Design review of the part built by this model. Coordinates are the model's own, in mm. A direction names the side the tool comes from. Round coordinates to 2 decimals unless told otherwise and drop trailing zeros. Order: outer loops, then holes, each group sorted by start corner. A loop starts at its lowest first (then second) coordinate and runs counter-clockwise, first axis right, second up. Notation, with made-up numbers: (11, 62.25) - (70, 62.25) arc R16 ccw to (70, 72.25) - close; hole circle Ø1 at (86.25, 35). An arc over 180 degrees is marked (long way). Write item = value, one per line.
from build123d import *

# Parameters (mm, degrees)
BOSS_EXTRUDE1_DEPTH        = 6.35
BOSS_EXTRUDE2_DEPTH        = 6.35
CUT_EXTRUDE2_REACH         = 178.705
SKETCH3_R                  = 25.4
SKETCH3_R_2                = 14.2875
F_6_CLEARANCE_HOLE1_D      = 3.6576
TAP_DRILL_FOR_10_32_TAP1_D = 4.0386


with BuildPart() as part:
    # Sketch1 → Boss-Extrude1 (new body)
    with BuildSketch(Plane(origin=(0, 0, 0), x_dir=(1, 0, 0), z_dir=(0, 1, 0))):
        with BuildLine():
            Line((-82.55, -50.8), (-10.295626201, -150.844517568))
            ThreePointArc((-10.295626201, -150.844517568), (0, -156.108787534), (10.295626201, -150.844517568))
            Line((10.295626201, -150.844517568), (82.55, -50.8))
            Line((82.55, -50.8), (82.55, 50.8))
            Line((82.55, 50.8), (-82.55, 50.8))
            Line((-82.55, 50.8), (-82.55, -50.8))
        make_face()
    extrude(amount=BOSS_EXTRUDE1_DEPTH)

    # Sketch4 → Boss-Extrude2 (add)
    with BuildSketch(Plane(origin=(0, 6.35, 0), x_dir=(1, 0, 0), z_dir=(0, 1, 0))):
        Polygon((-63.5, -77.176923077), (-63.5, -102.576923077), (-57.15, -102.576923077), (-57.15, -85.969230769), align=None)
        Polygon((57.15, -102.576923077), (63.5, -102.576923077), (63.5, -77.176923077), (57.15, -85.969230769), align=None)
    extrude(amount=-BOSS_EXTRUDE2_DEPTH)

    # Sketch3 → Cut-Extrude2 (cut, up to next)
    with BuildSketch(Plane(origin=(0, 6.35, 0), x_dir=(1, 0, 0), z_dir=(0, 1, 0)), mode=Mode.PRIVATE) as cut_extrude2_sk1:
        with Locations(Location((0, -50.8, 0), (0, 0, 270))):
            Circle(SKETCH3_R)
    cut_extrude2_tool1 = extrude(cut_extrude2_sk1.sketch, amount=-CUT_EXTRUDE2_REACH, mode=Mode.PRIVATE) & part.part
    # Sketch3 → Cut-Extrude2 (cut, up to next)
    with BuildSketch(Plane(origin=(0, 6.35, 0), x_dir=(1, 0, 0), z_dir=(0, 1, 0)), mode=Mode.PRIVATE) as cut_extrude2_sk2:
        with Locations(Location((0, -127, 0), (0, 0, 270))):
            Circle(SKETCH3_R_2)
    cut_extrude2_tool2 = extrude(cut_extrude2_sk2.sketch, amount=-CUT_EXTRUDE2_REACH, mode=Mode.PRIVATE) & part.part
    # Sketch3 → Cut-Extrude2 (cut, up to next)
    with BuildSketch(Plane(origin=(0, 6.35, 0), x_dir=(1, 0, 0), z_dir=(0, 1, 0)), mode=Mode.PRIVATE) as cut_extrude2_sk3:
        with BuildLine():
            Line((-58.367499255, 41.510492422), (-5.594504663, 9.034803443))
            ThreePointArc((-5.594504663, 9.034803443), (-3.988113518, 9.000996521), (-3.175, 10.386811021))
            Line((-3.175, 10.386811021), (-3.175, 42.8625))
            ThreePointArc((-3.175, 42.8625), (-3.639967985, 43.985032015), (-4.7625, 44.45))
            Line((-4.7625, 44.45), (-57.535494592, 44.45))
            ThreePointArc((-57.535494592, 44.45), (-59.062987354, 43.294844897), (-58.367499255, 41.510492422))
        make_face()
    cut_extrude2_tool3 = extrude(cut_extrude2_sk3.sketch, amount=-CUT_EXTRUDE2_REACH, mode=Mode.PRIVATE) & part.part
    # Sketch3 → Cut-Extrude2 (cut, up to next)
    with BuildSketch(Plane(origin=(0, 6.35, 0), x_dir=(1, 0, 0), z_dir=(0, 1, 0)), mode=Mode.PRIVATE) as cut_extrude2_sk4:
        with BuildLine():
            Line((-73.025, 36.505496672), (-73.025, 7.9375))
            ThreePointArc((-73.025, 7.9375), (-72.560032015, 6.814967985), (-71.4375, 6.35))
            Line((-71.4375, 6.35), (-25.014505408, 6.35))
            ThreePointArc((-25.014505408, 6.35), (-23.487012646, 7.505155103), (-24.182500745, 9.289507578))
            Line((-24.182500745, 9.289507578), (-70.605495337, 37.857504249))
            ThreePointArc((-70.605495337, 37.857504249), (-72.211886482, 37.891311171), (-73.025, 36.505496672))
        make_face()
    cut_extrude2_tool4 = extrude(cut_extrude2_sk4.sketch, amount=-CUT_EXTRUDE2_REACH, mode=Mode.PRIVATE) & part.part
    # Sketch3 → Cut-Extrude2 (cut, up to next)
    with BuildSketch(Plane(origin=(0, 6.35, 0), x_dir=(1, 0, 0), z_dir=(0, 1, 0)), mode=Mode.PRIVATE) as cut_extrude2_sk5:
        with BuildLine():
            Line((4.7625, 44.45), (57.535494592, 44.45))
            ThreePointArc((57.535494592, 44.45), (59.062987354, 43.294844897), (58.367499255, 41.510492422))
            Line((58.367499255, 41.510492422), (5.594504663, 9.034803443))
            ThreePointArc((5.594504663, 9.034803443), (3.988113518, 9.000996521), (3.175, 10.386811021))
            Line((3.175, 10.386811021), (3.175, 42.8625))
            ThreePointArc((3.175, 42.8625), (3.639967985, 43.985032015), (4.7625, 44.45))
        make_face()
    cut_extrude2_tool5 = extrude(cut_extrude2_sk5.sketch, amount=-CUT_EXTRUDE2_REACH, mode=Mode.PRIVATE) & part.part
    # Sketch3 → Cut-Extrude2 (cut, up to next)
    with BuildSketch(Plane(origin=(0, 6.35, 0), x_dir=(1, 0, 0), z_dir=(0, 1, 0)), mode=Mode.PRIVATE) as cut_extrude2_sk6:
        with BuildLine():
            Line((24.182500745, 9.289507578), (70.605495337, 37.857504249))
            ThreePointArc((70.605495337, 37.857504249), (72.211886482, 37.891311171), (73.025, 36.505496672))
            Line((73.025, 36.505496672), (73.025, 7.9375))
            ThreePointArc((73.025, 7.9375), (72.560032015, 6.814967985), (71.4375, 6.35))
            Line((71.4375, 6.35), (25.014505408, 6.35))
            ThreePointArc((25.014505408, 6.35), (23.487012646, 7.505155103), (24.182500745, 9.289507578))
        make_face()
    cut_extrude2_tool6 = extrude(cut_extrude2_sk6.sketch, amount=-CUT_EXTRUDE2_REACH, mode=Mode.PRIVATE) & part.part
    # Sketch3 → Cut-Extrude2 (cut, up to next)
    with BuildSketch(Plane(origin=(0, 6.35, 0), x_dir=(1, 0, 0), z_dir=(0, 1, 0)), mode=Mode.PRIVATE) as cut_extrude2_sk7:
        with BuildLine():
            Line((73.025, -36.505496672), (73.025, -7.9375))
            ThreePointArc((73.025, -7.9375), (72.560032015, -6.814967985), (71.4375, -6.35))
            Line((71.4375, -6.35), (25.014505408, -6.35))
            ThreePointArc((25.014505408, -6.35), (23.487012646, -7.505155103), (24.182500745, -9.289507578))
            Line((24.182500745, -9.289507578), (70.605495337, -37.857504249))
            ThreePointArc((70.605495337, -37.857504249), (72.211886482, -37.891311171), (73.025, -36.505496672))
        make_face()
    cut_extrude2_tool7 = extrude(cut_extrude2_sk7.sketch, amount=-CUT_EXTRUDE2_REACH, mode=Mode.PRIVATE) & part.part
    # Sketch3 → Cut-Extrude2 (cut, up to next)
    with BuildSketch(Plane(origin=(0, 6.35, 0), x_dir=(1, 0, 0), z_dir=(0, 1, 0)), mode=Mode.PRIVATE) as cut_extrude2_sk8:
        with BuildLine():
            Line((-24.182500745, -9.289507578), (-70.605495337, -37.857504249))
            ThreePointArc((-70.605495337, -37.857504249), (-72.211886482, -37.891311171), (-73.025, -36.505496672))
            Line((-73.025, -36.505496672), (-73.025, -7.9375))
            ThreePointArc((-73.025, -7.9375), (-72.560032015, -6.814967985), (-71.4375, -6.35))
            Line((-71.4375, -6.35), (-25.014505408, -6.35))
            ThreePointArc((-25.014505408, -6.35), (-23.487012646, -7.505155103), (-24.182500745, -9.289507578))
        make_face()
    cut_extrude2_tool8 = extrude(cut_extrude2_sk8.sketch, amount=-CUT_EXTRUDE2_REACH, mode=Mode.PRIVATE) & part.part
    # Sketch3 → Cut-Extrude2 (cut, up to next)
    with BuildSketch(Plane(origin=(0, 6.35, 0), x_dir=(1, 0, 0), z_dir=(0, 1, 0)), mode=Mode.PRIVATE) as cut_extrude2_sk9:
        with BuildLine():
            Line((-6.35, -85.142875899), (-6.35, -105.615701316))
            ThreePointArc((-6.35, -105.615701316), (-15.402705776, -110.864096399), (-21.066111407, -119.663128703))
            Line((-21.066111407, -119.663128703), (-68.507537692, -53.975))
            Line((-68.507537692, -53.975), (-34.780382402, -53.975))
            ThreePointArc((-34.780382402, -53.975), (-25.802833394, -74.336554843), (-6.35, -85.142875899))
        make_face()
    cut_extrude2_tool9 = extrude(cut_extrude2_sk9.sketch, amount=-CUT_EXTRUDE2_REACH, mode=Mode.PRIVATE) & part.part
    # Sketch3 → Cut-Extrude2 (cut, up to next)
    with BuildSketch(Plane(origin=(0, 6.35, 0), x_dir=(1, 0, 0), z_dir=(0, 1, 0)), mode=Mode.PRIVATE) as cut_extrude2_sk10:
        with BuildLine():
            Line((6.35, -85.142875899), (6.35, -105.615701316))
            ThreePointArc((6.35, -105.615701316), (15.402705776, -110.864096399), (21.066111407, -119.663128703))
            Line((21.066111407, -119.663128703), (68.507537692, -53.975))
            Line((68.507537692, -53.975), (34.780382402, -53.975))
            ThreePointArc((34.780382402, -53.975), (25.802833394, -74.336554843), (6.35, -85.142875899))
        make_face()
    cut_extrude2_tool10 = extrude(cut_extrude2_sk10.sketch, amount=-CUT_EXTRUDE2_REACH, mode=Mode.PRIVATE) & part.part
    # Sketch3 → Cut-Extrude2 (cut, up to next)
    with BuildSketch(Plane(origin=(0, 6.35, 0), x_dir=(1, 0, 0), z_dir=(0, 1, 0)), mode=Mode.PRIVATE) as cut_extrude2_sk11:
        with BuildLine():
            Line((-19.05, -21.527946348), (-19.05, 0))
            ThreePointArc((-19.05, 0), (0, 5.652946348), (19.05, 0))
            Line((19.05, 0), (19.05, -21.527946348))
            ThreePointArc((19.05, -21.527946348), (0, -15.875), (-19.05, -21.527946348))
        make_face()
    cut_extrude2_tool11 = extrude(cut_extrude2_sk11.sketch, amount=-CUT_EXTRUDE2_REACH, mode=Mode.PRIVATE) & part.part
    # Sketch3 → Cut-Extrude2 (cut, up to next)
    with BuildSketch(Plane(origin=(0, 6.35, 0), x_dir=(1, 0, 0), z_dir=(0, 1, 0)), mode=Mode.PRIVATE) as cut_extrude2_sk12:
        with BuildLine():
            Line((-57.535494592, -44.45), (-35.639286609, -44.45))
            ThreePointArc((-35.639286609, -44.45), (-34.646236712, -44.101050827), (-34.089752409, -43.207608696))
            ThreePointArc((-34.089752409, -43.207608696), (-30.993130541, -34.700885606), (-25.814130435, -27.275835936))
            ThreePointArc((-25.814130435, -27.275835936), (-25.507148617, -26.779893377), (-25.4, -26.206555752))
            Line((-25.4, -26.206555752), (-25.4, -24.063734098))
            ThreePointArc((-25.4, -24.063734098), (-26.213113518, -22.677919598), (-27.819504663, -22.71172652))
            Line((-27.819504663, -22.71172652), (-58.367499255, -41.510492422))
            ThreePointArc((-58.367499255, -41.510492422), (-59.062987354, -43.294844897), (-57.535494592, -44.45))
        make_face()
    cut_extrude2_tool12 = extrude(cut_extrude2_sk12.sketch, amount=-CUT_EXTRUDE2_REACH, mode=Mode.PRIVATE) & part.part
    # Sketch3 → Cut-Extrude2 (cut, up to next)
    with BuildSketch(Plane(origin=(0, 6.35, 0), x_dir=(1, 0, 0), z_dir=(0, 1, 0)), mode=Mode.PRIVATE) as cut_extrude2_sk13:
        with BuildLine():
            Line((25.4, -24.063734098), (25.4, -26.206555752))
            ThreePointArc((25.4, -26.206555752), (25.507148617, -26.779893377), (25.814130435, -27.275835936))
            ThreePointArc((25.814130435, -27.275835936), (30.993130541, -34.700885606), (34.089752409, -43.207608696))
            ThreePointArc((34.089752409, -43.207608696), (34.646236712, -44.101050827), (35.639286609, -44.45))
            Line((35.639286609, -44.45), (57.535494592, -44.45))
            ThreePointArc((57.535494592, -44.45), (59.062987354, -43.294844897), (58.367499255, -41.510492422))
            Line((58.367499255, -41.510492422), (27.819504663, -22.71172652))
            ThreePointArc((27.819504663, -22.71172652), (26.213113518, -22.677919598), (25.4, -24.063734098))
        make_face()
    cut_extrude2_tool13 = extrude(cut_extrude2_sk13.sketch, amount=-CUT_EXTRUDE2_REACH, mode=Mode.PRIVATE) & part.part
    add(cut_extrude2_tool1.solids().sort_by_distance((0, 6.35, 50.8))[0], mode=Mode.SUBTRACT)
    add(cut_extrude2_tool2.solids().sort_by_distance((0, 6.35, 127))[0], mode=Mode.SUBTRACT)
    add(cut_extrude2_tool3.solids().sort_by_distance((-23.016302, 6.35, -32.123089))[0], mode=Mode.SUBTRACT)
    add(cut_extrude2_tool4.solids().sort_by_distance((-55.316443, 6.35, -17.377083))[0], mode=Mode.SUBTRACT)
    add(cut_extrude2_tool5.solids().sort_by_distance((23.016302, 6.35, -32.123089))[0], mode=Mode.SUBTRACT)
    add(cut_extrude2_tool6.solids().sort_by_distance((55.316443, 6.35, -17.377083))[0], mode=Mode.SUBTRACT)
    add(cut_extrude2_tool7.solids().sort_by_distance((55.316443, 6.35, 17.377083))[0], mode=Mode.SUBTRACT)
    add(cut_extrude2_tool8.solids().sort_by_distance((-55.316443, 6.35, 17.377083))[0], mode=Mode.SUBTRACT)
    add(cut_extrude2_tool9.solids().sort_by_distance((-32.99022, 6.35, 82.3723))[0], mode=Mode.SUBTRACT)
    add(cut_extrude2_tool10.solids().sort_by_distance((32.99022, 6.35, 82.3723))[0], mode=Mode.SUBTRACT)
    add(cut_extrude2_tool11.solids().sort_by_distance((0, 6.35, 6.929783))[0], mode=Mode.SUBTRACT)
    add(cut_extrude2_tool12.solids().sort_by_distance((-40.378487, 6.35, 36.296551))[0], mode=Mode.SUBTRACT)
    add(cut_extrude2_tool13.solids().sort_by_distance((40.378487, 6.35, 36.296551))[0], mode=Mode.SUBTRACT)

    # #6 Clearance Hole1 (through all)
    with Locations(Plane(origin=(0, 6.35, 0), x_dir=(1, 0, 0), z_dir=(0, 1, 0))):
        with Locations((-79.375, -44.45), (-79.375, 3.175), (-69.85, 47.625), (-79.375, 34.925), (-38.1, 47.625), (0, 47.625), (38.1, 47.625), (69.85, 47.625), (79.375, 34.925), (79.375, 3.175), (79.375, -44.45)):
            Hole(F_6_CLEARANCE_HOLE1_D / 2)

    # Tap Drill for #10-32 Tap1 (through all)
    with Locations(Plane(origin=(0, 6.35, 0), x_dir=(1, 0, 0), z_dir=(0, 1, 0))):
        with Locations((-38.1, -50.8), (0, -88.9), (38.1, -50.8)):
            Hole(TAP_DRILL_FOR_10_32_TAP1_D / 2)


solid = part.part
Item 1: For faces 3 (the face through (-32.35, 3.22, -25.5)), 4 (the face through (-34.051, 3.131, 117.953)), list the 3-axis set-ups (+Z, -Z, +X, -X, +Y, -Y) from which the entire face can be reached by the end or side of a thin tool; tool diameter is ignored.
Data:
face_3 = +Y, -Y
face_4 = +Z, +Y, -Y
Item 2: Take a section at A-A, the plane z = 71. State the section outline as (x, y) points.
Data:
outline = (-67.96, 0) - (-56.21, 0) - (-56.21, 6.35) - (-67.96, 6.35) - close; (-28.49, 0) - (-15.4, 0) - (-15.4, 6.35) - (-28.49, 6.35) - close; (15.4, 0) - (28.49, 0) - (28.49, 6.35) - (15.4, 6.35) - close; (56.21, 0) - (67.96, 0) - (67.96, 6.35) - (56.21, 6.35) - close
Item 3: The part is to be moulded in two halves that separate along X. For faces 1 (the face through (-0.168, 3.131, 156.108)), 2 (the face through (49, 3, 6.35)), say which applies: +X half, -X half, draft (parallel to the pull), parting line (faces both ways), or undercut.
Data:
face_1 = parting line
face_2 = undercut
Item 4: Take a section at C-C, the plane z = 127. State the section outline as (x, y) points, and give its area (3 significant figures).
Data:
outline = (-27.52, 0) - (-14.29, 0) - (-14.29, 6.35) - (-27.52, 6.35) - close; (14.29, 0) - (27.52, 0) - (27.52, 6.35) - (14.29, 6.35) - close
area = 168 mm2
Item 5: For line 1 along Z through (x, y) = (-71.5, 5.25); line 2 along X through (y, z) = (2, -27) (3 decimals); line 3 along Z through (x, y) = (42.5, 4.5) (3 decimals), list the stretches that pass through material, from the lowest coordinate up. Write a range as [from, to].
Data:
line_1 = [-50.8, -48.41], [-46.84, -38.09], [-6.35, 6.35], [38.09, 66.1]
line_2 = [-82.55, -73.025], [-52.962, -34.788], [-3.175, 3.175], [34.788, 52.962], [73.025, 82.55]
line_3 = [-50.8, -44.45], [-31.746, -20.562], [-6.35, 6.35], [20.562, 31.746], [44.45, 53.975], [89.985, 106.254]
Item 6: Take a section at D-D, the plane y = 1. Count the separate pieces of the cut face and the enclosed holes in it, and give its area (3 significant figures).
Data:
separate_pieces = 1
enclosed_holes = 27
area = 12,900 mm2
Item 7: Insertion check: P1, Ø1, axis at y = 4, z = 118, coming from the -X side; P2, Ø1.9, axis at x = -56, y = 4.5, coming from the +Z side; P3, Ø6, axis at x = 79.375, z = -3.175, coming from the -Y side; P4, Ø1.5, axis at x = 21.5, y = 3.5, coming from the +Z side. Each pin has a flat end and moves straight along its axis. Give the tip position at first contact, or say it passes through.
Data:
P1 = -34.38
P2 = 88.88
P3 = 0
P4 = 136.37
Item 8: Take a section at B-B, the plane x = 43.5. State the section outline as (y, z) points (3 decimals).
Data:
outline = (0, -50.8) - (6.35, -50.8) - (6.35, -44.45) - (0, -44.45) - close; (0, -32.361) - (6.35, -32.361) - (6.35, -21.177) - (0, -21.177) - close; (0, -6.35) - (6.35, -6.35) - (6.35, 6.35) - (0, 6.35) - close; (0, 21.177) - (6.35, 21.177) - (6.35, 32.361) - (0, 32.361) - close; (0, 44.45) - (6.35, 44.45) - (6.35, 53.975) - (0, 53.975) - close; (0, 88.601) - (6.35, 88.601) - (6.35, 104.869) - (0, 104.869) - close
